Read the model definition and answer for the solid it produces. Units are mm, in the model's axes. Face numbers are marked on the shaded views. A direction names the side the tool comes from. Round coordinates to 2 decimals unless told otherwise and drop trailing zeros. Loops run counter-clockwise (first coordinate to the right, second up) from the corner with the lowest first, then second, coordinate; pieces in that order, holes last. Notation, with made-up numbers: M -15,78 L 30,78 A17 cw 30,94 Z; hole C 78.25,-25.75 d6. An arc over 180 degrees is marked long. Write each question's results on one line, items separated by ' | '.
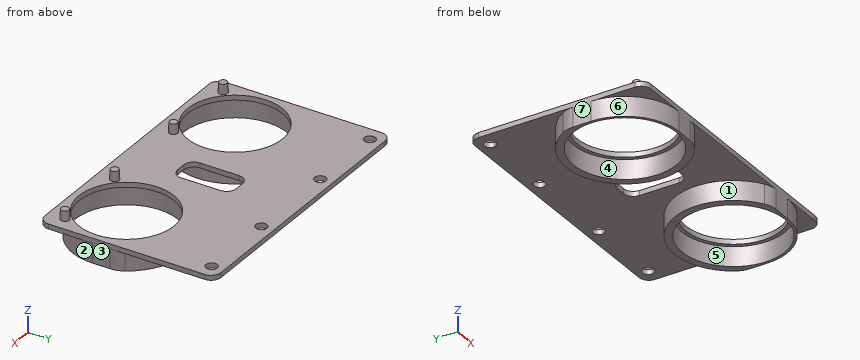
```python
from build123d import *

# Parameters (mm, degrees)
SKETCH_1_W                = 57
SKETCH_1_H                = 36
SKETCH_1_R                = 9.7
SKETCH_1_R_2              = 1.15
SKETCH_1_W_2              = 6
SKETCH_1_H_2              = 12
EXTRUDE_1_DEPTH           = 1
FILLET_1_R                = 2
FILLET_2_R                = 2
SKETCH_2_R                = 0.9
EXTRUDE_2_DEPTH           = 2
EXTRUDE_2_DRAFT           = 3
EXTRUDE_2_PROFILE_2_DEPTH = 2
EXTRUDE_2_PROFILE_2_DRAFT = 3
MIRROR_1_COPY_1_SKETCH_R  = 0.9
MIRROR_1_COPY_1_DEPTH     = 2
MIRROR_1_COPY_1_DRAFT     = 3
MIRROR_1_COPY_2_SKETCH_R  = 0.9
MIRROR_1_COPY_2_DEPTH     = 2
MIRROR_1_COPY_2_DRAFT     = 3
MIRROR_1_COPY_3_SKETCH_R  = 0.9
MIRROR_1_COPY_3_DEPTH     = 2
MIRROR_1_COPY_3_DRAFT     = 3
SKETCH_3_R                = 10.5
EXTRUDE_3_DEPTH           = 4
FILLET_3_R                = 5


with BuildPart() as part:
    # 草图1 → 凸台-拉伸1 (new body)
    with BuildSketch(Plane.XY):
        with Locations((0, 18)):
            Rectangle(SKETCH_1_W, SKETCH_1_H)
        with Locations((17.5, 11)):
            Circle(SKETCH_1_R, mode=Mode.SUBTRACT)
        with Locations(Location((-17.5, 11, 0), (0, 0, 180))):
            Circle(SKETCH_1_R, mode=Mode.SUBTRACT)
        with Locations((25.5, 33.5)):
            Circle(SKETCH_1_R_2, mode=Mode.SUBTRACT)
        with Locations((9.5, 33.5)):
            Circle(SKETCH_1_R_2, mode=Mode.SUBTRACT)
        with Locations(Location((-9.5, 33.5, 0), (0, 0, 180))):
            Circle(SKETCH_1_R_2, mode=Mode.SUBTRACT)
        with Locations(Location((-25.5, 33.5, 0), (0, 0, 180))):
            Circle(SKETCH_1_R_2, mode=Mode.SUBTRACT)
        with Locations((0, 17)):
            Rectangle(SKETCH_1_W_2, SKETCH_1_H_2, mode=Mode.SUBTRACT)
    extrude(amount=-EXTRUDE_1_DEPTH)

    # 圆角1
    fillet_1_edges = [part.edges().sort_by_distance(p)[0] for p in [
        (28.5, 0, -0.5),
        (-28.5, 0, -0.5),
        (-28.5, 36, -0.5),
        (28.5, 36, -0.5),
    ]]
    fillet(fillet_1_edges, radius=FILLET_1_R)

    # 圆角2
    fillet_2_edges = [part.edges().sort_by_distance(p)[0] for p in [
        (-3, 11, -0.5),
        (-3, 23, -0.5),
        (3, 23, -0.5),
        (3, 11, -0.5),
    ]]
    fillet(fillet_2_edges, radius=FILLET_2_R)


with BuildPart() as extrude_2_tool:
    # 草图2 → 凸台-拉伸2 (with draft: the straight prism first)
    with BuildSketch(Plane.XY):
        with Locations((-25.5, 3.5)):
            Circle(SKETCH_2_R)
    extrude(amount=EXTRUDE_2_DEPTH)
    # 凸台-拉伸2: the draft: its side faces are tilted about the plane it starts from
    extrude_2_sides = [extrude_2_tool.faces().sort_by_distance(p)[0] for p in [
        (-26.4, 3.5, 1),
    ]]
    draft(extrude_2_sides, Plane.XY, EXTRUDE_2_DRAFT)


with BuildPart() as part_1:
    add(part.part)

    # 凸台-拉伸2: add extrude_2_tool
    add(extrude_2_tool.part)


with BuildPart() as extrude_2_profile_2_tool:
    # 草图2 → 凸台-拉伸2 profile 2 (with draft: the straight prism first)
    with BuildSketch(Plane.XY):
        with Locations((-9.5, 3.5)):
            Circle(SKETCH_2_R)
    extrude(amount=EXTRUDE_2_PROFILE_2_DEPTH)
    # 凸台-拉伸2 profile 2: the draft: its side faces are tilted about the plane it starts from
    extrude_2_profile_2_sides = [extrude_2_profile_2_tool.faces().sort_by_distance(p)[0] for p in [
        (-10.4, 3.5, 1),
    ]]
    draft(extrude_2_profile_2_sides, Plane.XY, EXTRUDE_2_PROFILE_2_DRAFT)


with BuildPart() as part_2:
    add(part_1.part)

    # 凸台-拉伸2 profile 2: add extrude_2_profile_2_tool
    add(extrude_2_profile_2_tool.part)


with BuildPart() as mirror_1_copy_1_tool:
    # 镜向1 copy 1 sketch → 镜向1 copy 1 (with draft: the straight prism first)
    with BuildSketch(Plane(origin=(0, 0, 0), x_dir=(-1, 0, 0), z_dir=(0, 0, 1))):
        with Locations((-25.5, -3.5)):
            Circle(MIRROR_1_COPY_1_SKETCH_R)
    extrude(amount=MIRROR_1_COPY_1_DEPTH)
    # 镜向1 copy 1: the draft: its side faces are tilted about the plane it starts from
    mirror_1_copy_1_sides = [mirror_1_copy_1_tool.faces().sort_by_distance(p)[0] for p in [
        (26.4, 3.5, 1),
    ]]
    draft(mirror_1_copy_1_sides, Plane(origin=(0, 0, 0), x_dir=(-1, 0, 0), z_dir=(0, 0, 1)), MIRROR_1_COPY_1_DRAFT)


with BuildPart() as part_3:
    add(part_2.part)

    # 镜向1 copy 1: add mirror_1_copy_1_tool
    add(mirror_1_copy_1_tool.part)


with BuildPart() as mirror_1_copy_2_tool:
    # 镜向1 copy 2 sketch → 镜向1 copy 2 (with draft: the straight prism first)
    with BuildSketch(Plane(origin=(0, 0, 0), x_dir=(-1, 0, 0), z_dir=(0, 0, 1))):
        with Locations((-9.5, -3.5)):
            Circle(MIRROR_1_COPY_2_SKETCH_R)
    extrude(amount=MIRROR_1_COPY_2_DEPTH)
    # 镜向1 copy 2: the draft: its side faces are tilted about the plane it starts from
    mirror_1_copy_2_sides = [mirror_1_copy_2_tool.faces().sort_by_distance(p)[0] for p in [
        (10.4, 3.5, 1),
    ]]
    draft(mirror_1_copy_2_sides, Plane(origin=(0, 0, 0), x_dir=(-1, 0, 0), z_dir=(0, 0, 1)), MIRROR_1_COPY_2_DRAFT)


with BuildPart() as part_4:
    add(part_3.part)

    # 镜向1 copy 2: add mirror_1_copy_2_tool
    add(mirror_1_copy_2_tool.part)


with BuildPart() as mirror_1_copy_3_tool:
    # 镜向1 copy 3 sketch → 镜向1 copy 3 (with draft: the straight prism first)
    with BuildSketch(Plane(origin=(0, 0, 0), x_dir=(-1, 0, 0), z_dir=(0, 0, 1))):
        with Locations((-9.5, -3.5)):
            Circle(MIRROR_1_COPY_3_SKETCH_R)
    extrude(amount=MIRROR_1_COPY_3_DEPTH)
    # 镜向1 copy 3: the draft: its side faces are tilted about the plane it starts from
    mirror_1_copy_3_sides = [mirror_1_copy_3_tool.faces().sort_by_distance(p)[0] for p in [
        (10.4, 3.5, 1),
    ]]
    draft(mirror_1_copy_3_sides, Plane(origin=(0, 0, 0), x_dir=(-1, 0, 0), z_dir=(0, 0, 1)), MIRROR_1_COPY_3_DRAFT)


with BuildPart() as part_5:
    add(part_4.part)

    # 镜向1 copy 3: add mirror_1_copy_3_tool
    add(mirror_1_copy_3_tool.part)

    # 草图3 → 凸台-拉伸3 (add)
    # profile 1 of 2: a face of its own
    with BuildSketch(Plane(origin=(0, 0, -1), x_dir=(-1, 0, 0), z_dir=(0, 0, -1))):
        with BuildLine():
            ThreePointArc((-12.704168477, 0), (-9.014718626, 19.485281374), (-28.5, 15.795831523))
            Line((-28.5, 15.795831523), (-28.5, 11))
            ThreePointArc((-28.5, 11), (-25.278174593, 3.221825407), (-17.5, 0))
            Line((-17.5, 0), (-12.704168477, 0))
        make_face()
        with Locations((-17.5, 11)):
            Circle(SKETCH_3_R, mode=Mode.SUBTRACT)
    # profile 2 of 2: a face of its own
    with BuildSketch(Plane(origin=(0, 0, -1), x_dir=(-1, 0, 0), z_dir=(0, 0, -1))):
        with BuildLine():
            ThreePointArc((28.5, 15.795831523), (9.014718626, 19.485281374), (12.704168477, 0))
            Line((12.704168477, 0), (17.5, 0))
            ThreePointArc((17.5, 0), (25.278174593, 3.221825407), (28.5, 11))
            Line((28.5, 11), (28.5, 15.795831523))
        make_face()
        with Locations((17.5, 11)):
            Circle(SKETCH_3_R, mode=Mode.SUBTRACT)
    extrude(amount=EXTRUDE_3_DEPTH)

    # 圆角3
    fillet_3_edges = [part_5.edges().sort_by_distance(p)[0] for p in [
        (28.5, 15.795831523, -3),
        (12.704168477, 0, -3),
        (-12.704168477, 0, -3),
        (-28.5, 15.795831523, -3),
    ]]
    fillet(fillet_3_edges, radius=FILLET_3_R)


solid = part_5.part
```
1. Find section A-A, the plane z = -4. Give the vertices of the cut face in (x, y), then the cut area to 3 significant figures.
Completed:
outline: M -28.5,11 A11 ccw -17.5,0 L -13.89,0 A5 ccw -11.32,0.71 A12 ccw long -27.79,17.18 A5 ccw -28.5,14.61 Z; M 11.32,0.71 A5 ccw 13.89,0 L 17.5,0 A11 ccw 28.5,11 L 28.5,14.61 A5 ccw 27.79,17.18 A12 ccw long Z; hole C -17.5,11 d21; hole C 17.5,11 d21 | area: 163 mm2
2. Which of the six approach directions +Z, -Z, +X, -X, +Y, -Y give full straight-line access (tool end or side, diameter ignored) to the marked faces 1, 2 and 3?
Completed:
face 1: -Z | face 2: -Z, +X, -Y | face 3: +Z, -Z, +X, +Y, -Y
3. Find section B-B, the plane x = 9.5. Give the vertices of the cut face in (y, z), then the cut area to 3 significant figures.
Completed:
outline: M 0,-1 L 2.06,-1 L 2.06,-5 L 4.2,-5 L 4.2,-1 L 5.51,-1 L 5.51,0 L 4.4,0 L 4.3,2 L 2.7,2 L 2.6,0 L 0,0 Z; M 16.49,-1 L 17.8,-1 L 17.8,-5 L 19.94,-5 L 19.94,-1 L 32.35,-1 L 32.35,0 L 16.49,0 Z; M 34.65,-1 L 36,-1 L 36,0 L 34.65,0 Z | area: 43.3 mm2
4. Find section D-D, the plane y = 31. Give the vertices of the cut face in (x, z).
Completed:
outline: M -28.5,-1 L 28.5,-1 L 28.5,0 L -28.5,0 Z
5. Given P1, Ø4, axis at y = 9.5, z = -2.5, coming from the +X side; P2, Ø2.5, axis at x = 9.5, y = 33.5, coming from the -Z side; P3, Ø3.5, axis at x = -25.5, y = 33.5, coming from the +Z side; P4, Ø1, axis at x = -8, z = -4, coming from the +Y side, each flat-ended and moving along its own axis, determine where each tip first touches the part or whether it passes through.
Completed:
P1: stops at x = 28.5 | P2: stops at z = -1 | P3: stops at z = 0 | P4: stops at y = 18.94
6. Determine the mould class of the marked faces 4, 5, 6 and 7 for opening direction Y: released by +Y, released by -Y, zero draft, split by the parting line, or undercut.
Completed:
face 4: undercut | face 5: undercut | face 6: released by -Y | face 7: zero draft
7. Find the intervals of material crossed by L1, parallel to Y at x = -25.5, z = -0.3; L2, parallel to Z at x = -22, y = 20; L3, parallel to Y at x = 17.5, z = -3.9, in increasing order.
Completed:
L1: y = 0 to 5.51, 16.49 to 32.35, 34.65 to 36 | L2: z = -1 to 0 | L3: y = 0 to 0.5, 21.5 to 23
8. Find section C-C, the plane x = -21. Give the vertices of the cut face in (y, z).
Completed:
outline: M 0,-1 L 0.57,-1 L 0.57,-5 L 1.1,-5 L 1.1,-1 L 1.95,-1 L 1.95,0 L 0,0 Z; M 20.05,-1 L 20.9,-1 L 20.9,-5 L 22.48,-5 L 22.48,-1 L 36,-1 L 36,0 L 20.05,0 Z
